Geometry check sheet. Reference: the model listing, model coordinates, mm. Face numbers are marked on the shaded views. A direction names the side the tool comes from. Give positions to 0.01 mm unless a question says otherwise; leave off trailing zeros. Write each loop counter-clockwise with the first axis right and the second up, starting at its lowest first coordinate (ties: lowest second). Pieces come first, ordered by that corner, then holes.
(1) Depth check by flat-ended pin: P1, Ø5, axis at x = 2, z = 1.5, coming from the -Y side; P2, Ø1.5, axis at x = 2, y = 4, coming from the +Z side; P3, Ø3, axis at x = -3.5, y = 2, coming from the +Z side; P4, Ø3, axis at x = 0, z = 0, coming from the +Y side. Enter the tip coordinate at first touch or a pass-through.
(2) Thickness scan on line 1 along X through (y, z) = (2.85, 0); line 2 along Y through (x, z) = (-0.5, 4.5); line 3 along X through (y, z) = (5.75, 2.25). Record the ranges inside material, lowest first.
(3) Tool access check on the marked faces 1, 2 and 3. Record the directions out of +Z, -Z, +X, -X, +Y, -Y that give a thin tool (end or side, any length) a straight path to the whole face; none if there is none.
(4) Cross-section at D-D (z = -2.75). Record the boundary of the cut face in (x, y), and give its area (3 significant figures).
(5) Cross-section at B-B (z = 0). Record the boundary of the cut face in (x, y).
(6) Cross-section at A-A (x = 0). Record the boundary of the cut face in (y, z), and give its area (3 significant figures).
(7) Mould release check, pull along X, two halves, no side actions. Record for the marked faces 4, 5 and 6: +X half, -X half, draft (parallel to the pull), parting line (faces both ways), or undercut.
(8) Cross-section at C-C (y = 2). Record the boundary of the cut face in (x, z), and give its area (3 significant figures).
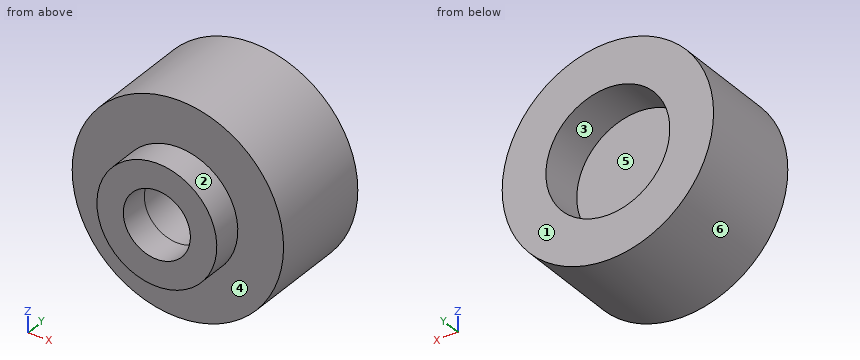
```python
from build123d import *

# Parameters (mm, degrees)
CROQUIS1_R              = 2.95
CROQUIS1_R_2            = 1.65
SALIENTE_EXTRUIR1_DEPTH = 1.5
CROQUIS2_R              = 5.2
SALIENTE_EXTRUIR2_DEPTH = 5.3
CROQUIS3_R              = 3.05
CORTAR_EXTRUIR1_DEPTH   = 2.3
CROQUIS4_R              = 1.65
CORTAR_EXTRUIR2_DEPTH   = 4.6
SALIENTE_EXTRUIR3_START = 0.1
CROQUIS5_R              = 3.05
SALIENTE_EXTRUIR3_DEPTH = 0.1


with BuildPart() as part:
    # Croquis1 → Saliente-Extruir1 (new body)
    with BuildSketch(Plane(origin=(0, 0, 0), x_dir=(1, 0, 0), z_dir=(0, 1, 0))):
        with Locations(Location((0, 0, 0), (0, 0, 270))):
            Circle(CROQUIS1_R)
        with Locations(Location((0, 0, 0), (0, 0, 270))):
            Circle(CROQUIS1_R_2, mode=Mode.SUBTRACT)
    extrude(amount=SALIENTE_EXTRUIR1_DEPTH)

    # Croquis2 → Saliente-Extruir2 (add)
    with BuildSketch(Plane(origin=(0, 1.5, 0), x_dir=(1, 0, 0), z_dir=(0, 1, 0))):
        with Locations(Location((0, 0, 0), (0, 0, 270))):
            Circle(CROQUIS2_R)
    extrude(amount=SALIENTE_EXTRUIR2_DEPTH)

    # Croquis3 → Cortar-Extruir1 (cut)
    with BuildSketch(Plane(origin=(0, 6.8, 0), x_dir=(1, 0, 0), z_dir=(0, 1, 0))):
        with Locations(Location((0, 0, 0), (0, 0, 270))):
            Circle(CROQUIS3_R)
    extrude(amount=-CORTAR_EXTRUIR1_DEPTH, mode=Mode.SUBTRACT)

    # Croquis4 → Cortar-Extruir2 (cut)
    with BuildSketch(Plane.XZ):
        with Locations(Location((0, 0, 0), (0, 0, 90))):
            Circle(CROQUIS4_R)
    extrude(amount=-CORTAR_EXTRUIR2_DEPTH, mode=Mode.SUBTRACT)

    # Croquis5 → Saliente-Extruir3 (add)
    with BuildSketch(Plane(origin=(0, 4.5, 0), x_dir=(1, 0, 0), z_dir=(0, 1, 0)).offset(SALIENTE_EXTRUIR3_START)):
        with Locations(Location((0, 0, 0), (0, 0, 270))):
            Circle(CROQUIS5_R)
    extrude(amount=-SALIENTE_EXTRUIR3_DEPTH)


solid = part.part
```
Reply:
1. P1: stops at y = 0
1. P2: stops at z = 5.05
1. P3: stops at z = 4.8
1. P4: stops at y = 4.6
2. line 1: x = -5.2 to -1.65, 1.65 to 5.2
2. line 2: y = 1.5 to 6.8
2. line 3: x = -4.69 to -2.06, 2.06 to 4.69
3. face 1: +Z, -Z, +X, -X, +Y
3. face 2: -Y
3. face 3: +Y
4. outline: (-4.41, 1.5) - (-1.07, 1.5) - (-1.07, 0) - (1.07, 0) - (1.07, 1.5) - (4.41, 1.5) - (4.41, 6.8) - (1.32, 6.8) - (1.32, 4.6) - (-1.32, 4.6) - (-1.32, 6.8) - (-4.41, 6.8) - close
4. area: 44.2 mm2
5. outline: (-5.2, 1.5) - (-2.95, 1.5) - (-2.95, 0) - (-1.65, 0) - (-1.65, 4.5) - (1.65, 4.5) - (1.65, 0) - (2.95, 0) - (2.95, 1.5) - (5.2, 1.5) - (5.2, 6.8) - (3.05, 6.8) - (3.05, 4.6) - (-3.05, 4.6) - (-3.05, 6.8) - (-5.2, 6.8) - close
6. outline: (0, -2.95) - (1.5, -2.95) - (1.5, -5.2) - (6.8, -5.2) - (6.8, -3.05) - (4.6, -3.05) - (4.6, 3.05) - (6.8, 3.05) - (6.8, 5.2) - (1.5, 5.2) - (1.5, 2.95) - (0, 2.95) - (0, 1.65) - (4.5, 1.65) - (4.5, -1.65) - (0, -1.65) - close
6. area: 35.7 mm2
7. face 4: draft
7. face 5: undercut
7. face 6: parting line
8. outline: circle Ø10.4 at (0, 0); hole circle Ø3.3 at (0, 0)
8. area: 76.4 mm2
